```python
from build123d import *

# Parameters (mm, degrees)
F1_DEPTH      = 30
F2_R          = 1.5
F3_R          = 1.5
F4_DEPTH      = 25
F4_DEPTH_BACK = 25
F5_SIZE       = 2


# Not quite as in the source:
# - a feature names something its author has since deleted; it is built from what else it names


with BuildPart() as f1:
    # F0 (on Top) → F1 (new body)
    with BuildSketch(Plane.XY):
        with BuildLine():
            Line((-5, 40), (-5, 0))
            ThreePointArc((-5, 0), (-14.8093771881, -7.1355992743), (-18.5778072009, 4.3943440499))
            ThreePointArc((-18.5778072009, 4.3943440499), (-19.1389615845, 7.8850611335), (-22.6296786681, 7.3239067498))
            ThreePointArc((-22.6296786681, 7.3239067498), (-16.3489619801, -11.8926654572), (0, 0))
            Line((0, 0), (0, 40))
            Line((0, 40), (-5, 40))
        make_face()
    extrude(amount=F1_DEPTH)

    # F2
    f2_edges = [f1.edges().sort_by_distance(p)[0] for p in [
        (-5, 40, 15),
        (0, 40, 15),
        (-16.348962, -11.892665, 0),
        (-16.348962, -11.892665, 30),
        (0, 20, 0),
        (-14.809377, -7.135599, 0),
        (-14.809377, -7.135599, 30),
        (-5, 20, 0),
        (-18.577807, 4.394344, 15),
        (-5, 20, 30),
        (-2.5, 40, 0),
        (0, 0, 15),
        (-22.629679, 7.323907, 15),
        (-2.5, 40, 30),
        (0, 20, 30),
        (-19.138962, 7.885061, 0),
        (-19.138962, 7.885061, 30),
    ]]
    fillet(f2_edges, radius=F2_R)

    # F3 (on face) → F4 (cut, two sides)
    with BuildSketch(Plane(origin=(-5, 0, 0), x_dir=(0, -1, 0), z_dir=(-1, 0, 0))) as f4_sk:
        with Locations((-23.5, 15)):
            Circle(F3_R)
        with Locations((-32.419529755, 23.0275767795)):
            Circle(F3_R)
        with Locations((-32.419529755, 6.9724232205)):
            Circle(F3_R)
    extrude(amount=F4_DEPTH, mode=Mode.SUBTRACT)
    extrude(f4_sk.sketch, amount=-F4_DEPTH_BACK, mode=Mode.SUBTRACT)

    # F5
    f5_edges = [f1.edges().sort_by_distance(p)[0] for p in [
        (-5, 33.91953, 6.972423),
        (-5, 33.91953, 23.027577),
        (-5, 25, 15),
    ]]
    chamfer(f5_edges, length=F5_SIZE)


solid = f1.part
```
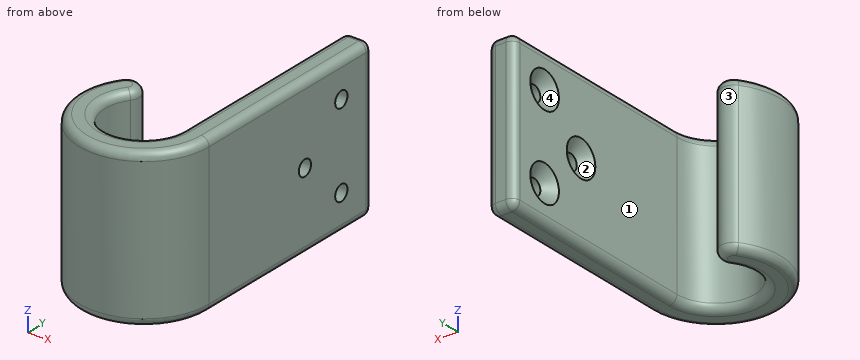
For this review, take the finished solid that the model builds, in its own axes (mm). Face numbers are marked on the shaded views. A direction names the side the tool comes from. Coordinates: 2 decimals unless noted, no trailing zeros. Write each loop counter-clockwise with the first axis right and the second up, starting at its lowest first coordinate (ties: lowest second). Pieces come first, ordered by that corner, then holes.
(1) Add section C-C on y = 16.5. Give the boundary of the cut face in (x, z), then the cut area to 3 significant figures.
(2) Add section B-B on z = 15. Give the boundary of the cut face in (x, y), then the cut area to 3 significant figures.
(3) Wall thickness on probe 1 along Z at (x, y) = (-1.8, 23.5); probe 2 along X at (y, z) = (13.5, 12.5); probe 3 along Z at (x, y) = (-1.75, 24): over which ranges is each line inside the solid? List them lowest first.
(4) Tool access review of the marked faces 1 and 2: name each direction out of +Z, -Z, +X, -X, +Y, -Y from which nothing blocks a thin tool from reaching the whole face with its end or side.
(5) Add section A-A on y = 23.5. Give the boundary of the cut face in (x, z), then the cut area to 3 significant figures.
(6) Add section D-D on y = 32. Count the separate pieces of the cut face and the enclosed holes in it, then the cut area to 3 significant figures.
(7) For pin 1 Ø6 at (x, z) = (-6.5, 9.5) entering from -Y; pin 2 Ø1.5 at (y, z) = (13.5, 19) entering from -X; pin 3 Ø5 at (x, z) = (-9.5, 13.5) entering from +Y, all flat-tipped, find the tip position at first contact; note any pin that passes through.
(8) The part is to be moulded in two halves that separate along Z. For the marked faces 3 and 4, say which applies: +Z half, -Z half, draft (parallel to the pull), parting line (faces both ways), or undercut.
Answer sheet:
1. outline: (-5, 1.5) arc R1.5 ccw to (-3.5, 0) - (-1.5, 0) arc R1.5 ccw to (0, 1.5) - (0, 28.5) arc R1.5 ccw to (-1.5, 30) - (-3.5, 30) arc R1.5 ccw to (-5, 28.5) - close
1. area: 148 mm2
2. outline: (-22.63, 7.32) arc R12.5 ccw (long way) to (0, 0) - (0, 22) - (-3, 22) - (-5, 20) - (-5, 0) arc R7.5 cw (long way) to (-18.58, 4.39) arc R2.5 ccw to start; (-5, 27) - (-3, 25) - (0, 25) - (0, 38.5) arc R1.5 ccw to (-1.5, 40) - (-3.5, 40) arc R1.5 ccw to (-5, 38.5) - close
2. area: 378 mm2
3. probe 1: z = 0 to 13.5, 16.5 to 30
3. probe 2: x = -5 to 0
3. probe 3: z = 0 to 13.59, 16.41 to 30
4. face 1: +Z, -Z, +Y
4. face 2: -X
5. outline: (-5, 1.5) arc R1.5 ccw to (-3.5, 0) - (-1.5, 0) arc R1.5 ccw to (0, 1.5) - (0, 13.5) - (-3, 13.5) - (-5, 11.5) - close; (-5, 18.5) - (-3, 16.5) - (0, 16.5) - (0, 28.5) arc R1.5 ccw to (-1.5, 30) - (-3.5, 30) arc R1.5 ccw to (-5, 28.5) - close
5. area: 129 mm2
6. separate pieces: 3
6. enclosed holes: 0
6. area: 111 mm2
7. pin 1: stops at y = -12.13
7. pin 2: stops at x = -5
7. pin 3: stops at y = -5.1
8. face 3: draft
8. face 4: undercut
